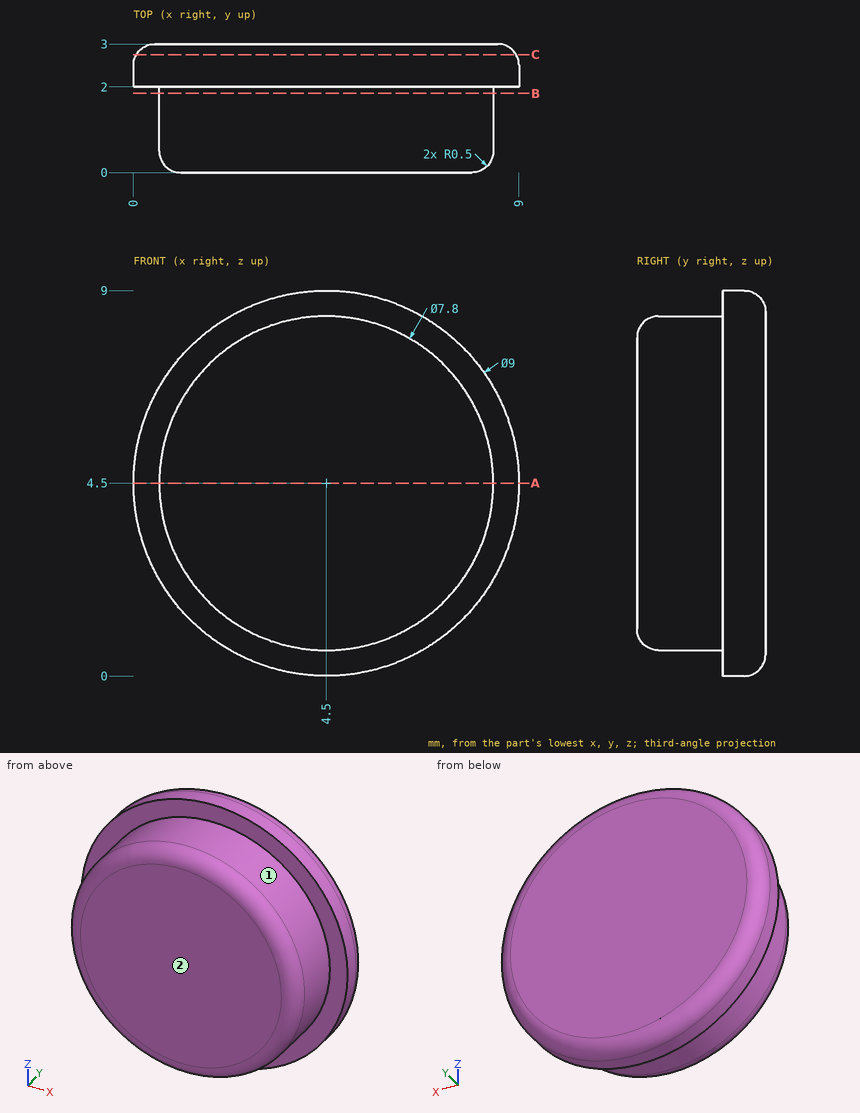
Check sheet for the drawn part. Datum: minimum x, y, z corner. Units: mm. A direction names the side the tool comes from. Give positions to 0.01 mm unless a question says otherwise; leave off trailing zeros. Loops run counter-clockwise (first coordinate to the right, second up) from the corner with the lowest first, then second, coordinate; pieces in that order, holes last.
1) Thickness scan on line 1 along X through (y, z) = (0.65, 6.5); line 2 along Z through (x, y) = (2.75, 2.5); line 3 along Y through (x, z) = (1, 3.75). Record the ranges inside material, lowest first.
2) Set-up check for the marked faces 1 and 2: record each of +Z, -Z, +X, -X, +Y, -Y from which the full face is reachable in a straight line by a thin tool's end or side.
3) Sectioned sample at A-A, the plane z = 4.5. Enter the section's corners in (x, y).
4) Sectioned sample at B-B, the plane y = 1.85. Enter the section's corners in (x, z), then the cut area to 3 significant figures.
5) Depth check by flat-ended pin: pin 1 Ø1 at (y, z) = (1, 5.5) entering from +X. Enter the tip coordinate at first touch or a pass-through.
6) Sectioned sample at C-C, the plane y = 2.75. Enter the section's corners in (x, z), then the cut area to 3 significant figures.
Answers:
1. line 1: x = 1.15 to 7.85
1. line 2: z = 0.35 to 8.65
1. line 3: y = 0.03 to 3
2. face 1: -Y
2. face 2: +Z, -Z, +X, -X, -Y
3. outline: (0, 2) - (0.6, 2) - (0.6, 0.5) arc R0.5 ccw to (1.1, 0) - (7.9, 0) arc R0.5 ccw to (8.4, 0.5) - (8.4, 2) - (9, 2) - (9, 2.5) arc R0.5 ccw to (8.5, 3) - (0.5, 3) arc R0.5 ccw to (0, 2.5) - close
4. outline: circle Ø7.8 at (4.5, 4.5)
4. area: 47.8 mm2
5. pin 1: stops at x = 8.37
6. outline: circle Ø8.87 at (4.5, 4.5)
6. area: 61.7 mm2
